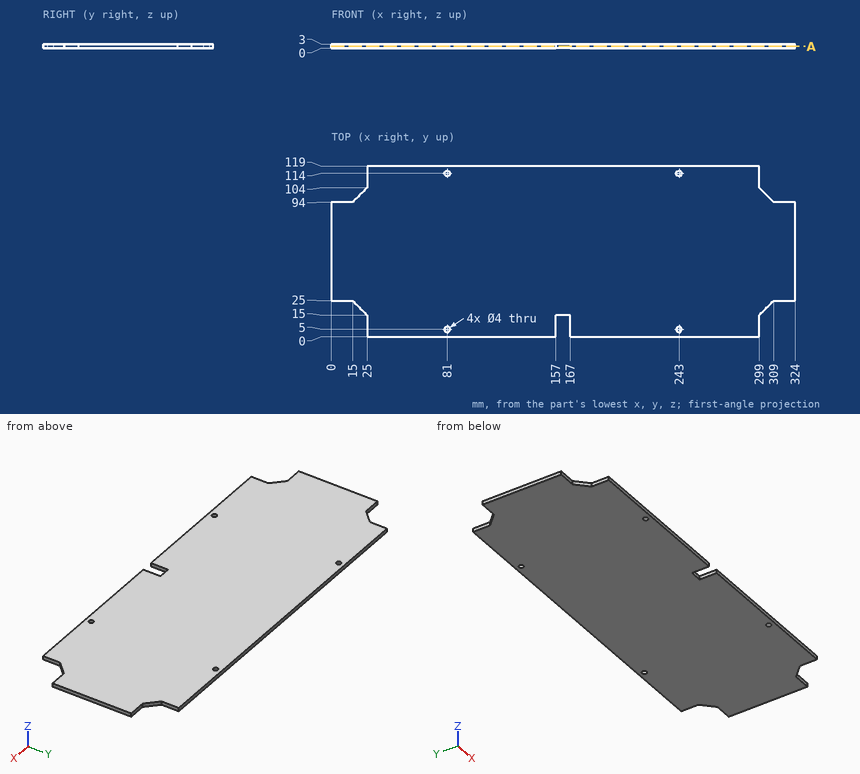
Verification items for this drawing (mm, ordinates from the low corner). Give positions to 0.01 mm unless a question says otherwise; leave off trailing zeros. Order: outer loops, then holes, each group sorted by start corner. A loop starts at its lowest first (then second) coordinate and runs counter-clockwise, first axis right, second up.
1) Cross-section at A-A (z = 1.3). Record the boundary of the cut face in (x, y).
Results are:
outline: (0, 25) - (15, 25) - (25, 15) - (25, 0) - (157, 0) - (157, 15) - (167, 15) - (167, 0) - (299, 0) - (299, 15) - (309, 25) - (324, 25) - (324, 94) - (309, 94) - (299, 104) - (299, 119) - (25, 119) - (25, 104) - (15, 94) - (0, 94) - close; hole circle Ø4 at (81, 5); hole circle Ø4 at (81, 114); hole circle Ø4 at (243, 5); hole circle Ø4 at (243, 114)
2) Material ranges on probe 1 along Y at (x, z) = (81, 1.3); probe 2 along X at (y, z) = (114.5, 1.75); probe 3 along Y at (x, z) = (79.5, 2.6), recorded low to high.
Results are:
probe 1: y = 0 to 3, 7 to 112, 116 to 119
probe 2: x = 25 to 79.06, 82.94 to 241.06, 244.94 to 299
probe 3: y = 0 to 3.68, 6.32 to 112.68, 115.32 to 119
3) Gauge pin test, flat ends, axial feed: pin 1 (0.9 mm diameter, centred on x = 317, z = 1.5, fed in from -Y); pin 2 (4.5 mm diameter, centred on x = 243, y = 114, fed in from -Z); pin 3 (1 mm diameter, centred on y = 99, z = 1.5, fed in from -X); pin 4 (1.5 mm diameter, centred on x = 5, z = 2, fed in from +Y). Record the tip position at first contact, or that the pin passes through.
Results are:
pin 1: stops at y = 25
pin 2: stops at z = 0
pin 3: stops at x = 19.5
pin 4: stops at y = 94
